from build123d import *

# Parameters (mm, degrees)
SKETCH2_R          = 6.57
CUT_EXTRUDE1_DEPTH = 10.189570175
SKETCH3_R          = 2.9
CUT_EXTRUDE2_DEPTH = 3.28
SKETCH4_R          = 0.9
CUT_EXTRUDE3_DEPTH = 11.034288305


with BuildPart() as part:
    # Sketch1 → Revolve1 (revolve)
    with BuildSketch(Plane.XY, mode=Mode.PRIVATE) as revolve1_sk:
        Polygon((0, 5.22), (0, 1), (2.72, 1), (2.72, 0.42), (4.45, 0.42), (4.45, 0), (6.07, 0), (6.07, 1.94), (2.4, 1.94), (2.4, 5.22), align=None)
    revolve(revolve1_sk.sketch.rotate(Axis((0, 5.22, 0), (0, -1, 0)), 180), axis=Axis((0, 5.22, 0), (0, -1, 0)))

    # Sketch2 → Cut-Extrude1 (cut, through all)
    with BuildSketch(Plane(origin=(0, 1.94, 0), x_dir=(1, 0, 0), z_dir=(0, 1, 0))):
        Circle(SKETCH2_R)
        Polygon((0, 6.07), (-0.459966954, 5.550975626), (-0.999089163, 5.987213112), (-1.367354163, 5.399559481), (-1.970925778, 5.741110657), (-2.237443515, 5.100857429), (-2.889000676, 5.33840567), (-3.046501241, 4.663017284), (-3.728271166, 4.790082892), (-3.772458354, 4.097982182), (-4.465844138, 4.11109914), (-4.395512637, 3.42116481), (-5.081600523, 3.31997532), (-4.898668794, 2.651026979), (-5.558744093, 2.438291228), (-5.268202036, 1.808576043), (-5.884259614, 1.490096907), (-5.49403246, 0.916791868), (-6.049267873, 0.501256627), (-5.57, 0), (-6.049267873, -0.501256627), (-5.49403246, -0.916791868), (-5.884259614, -1.490096907), (-5.268202036, -1.808576043), (-5.558744093, -2.438291228), (-4.898668794, -2.651026979), (-5.081600523, -3.31997532), (-4.395512637, -3.42116481), (-4.465844138, -4.11109914), (-3.772458354, -4.097982182), (-3.728271166, -4.790082892), (-3.046501241, -4.663017284), (-2.889000676, -5.33840567), (-2.237443515, -5.100857429), (-1.970925778, -5.741110657), (-1.367354163, -5.399559481), (-0.999089163, -5.987213112), (-0.459966954, -5.550975626), (0, -6.07), (0.459966954, -5.550975626), (0.999089163, -5.987213112), (1.367354163, -5.399559481), (1.970925778, -5.741110657), (2.237443515, -5.100857429), (2.889000676, -5.33840567), (3.046501241, -4.663017284), (3.728271166, -4.790082892), (3.772458354, -4.097982182), (4.465844138, -4.11109914), (4.395512637, -3.42116481), (5.081600523, -3.31997532), (4.898668794, -2.651026979), (5.558744093, -2.438291228), (5.268202036, -1.808576043), (5.884259614, -1.490096907), (5.49403246, -0.916791868), (6.049267873, -0.501256627), (5.57, 0), (6.049267873, 0.501256627), (5.49403246, 0.916791868), (5.884259614, 1.490096907), (5.268202036, 1.808576043), (5.558744093, 2.438291228), (4.898668794, 2.651026979), (5.081600523, 3.31997532), (4.395512637, 3.42116481), (4.465844138, 4.11109914), (3.772458354, 4.097982182), (3.728271166, 4.790082892), (3.046501241, 4.663017284), (2.889000676, 5.33840567), (2.237443515, 5.100857429), (1.970925778, 5.741110657), (1.367354163, 5.399559481), (0.999089163, 5.987213112), (0.459966954, 5.550975626), align=None, mode=Mode.SUBTRACT)
    extrude(amount=-CUT_EXTRUDE1_DEPTH, mode=Mode.SUBTRACT)

    # Sketch3 → Cut-Extrude2 (cut)
    with BuildSketch(Plane(origin=(0, 5.22, 0), x_dir=(1, 0, 0), z_dir=(0, 1, 0))):
        Circle(SKETCH3_R)
        Polygon((0, 2.4), (-0.463525492, 1.426584774), (-1.410684606, 1.941640786), (-1.213525492, 0.881677878), (-2.282535639, 0.741640786), (-1.5, 0), (-2.282535639, -0.741640786), (-1.213525492, -0.881677878), (-1.410684606, -1.941640786), (-0.463525492, -1.426584774), (0, -2.4), (0.463525492, -1.426584774), (1.410684606, -1.941640786), (1.213525492, -0.881677878), (2.282535639, -0.741640786), (1.5, 0), (2.282535639, 0.741640786), (1.213525492, 0.881677878), (1.410684606, 1.941640786), (0.463525492, 1.426584774), align=None, mode=Mode.SUBTRACT)
    extrude(amount=-CUT_EXTRUDE2_DEPTH, mode=Mode.SUBTRACT)

    # Sketch4 → Cut-Extrude3 (cut, through all)
    with BuildSketch(Plane(origin=(0, 5.22, 0), x_dir=(1, 0, 0), z_dir=(0, 1, 0))):
        with Locations(Location((0, 0, 0), (0, 0, 180))):
            Circle(SKETCH4_R)
    extrude(amount=-CUT_EXTRUDE3_DEPTH, mode=Mode.SUBTRACT)


solid = part.part
Design review of the part built by this model. Coordinates are the model's own, in mm. A direction names the side the tool comes from. Round coordinates to 2 decimals unless told otherwise and drop trailing zeros. Loops run counter-clockwise (first coordinate to the right, second up) from the corner with the lowest first, then second, coordinate; pieces in that order, holes last. Notation, with made-up numbers: (24, 74) - (41, 74) arc R25 ccw to (41, 92) - close; hole circle Ø11 at (-23, 75). An arc over 180 degrees is marked (long way). One line per item, written item: value. Start each with the question number.
1) Consider section D-D on x = 4.25. Give the boundary of the cut face in (y, z), then the cut area to 3 significant figures.
2) For faces 1 (the flat face through (0.93, 3.6, 1.68)), 2 (the flat face through (1.313, 3.603, 1.419)), 3 (the flat face through (0.235, 3.603, -1.906)), list the 3-axis set-ups (+Z, -Z, +X, -X, +Y, -Y) from which the entire face can be reached by the end or side of a thin tool; tool diameter is ignored.
3) To check wall thickness, follow L1, parallel to Y at x = -1.25, z = 1.25; L2, parallel to X at y = 1.05, z = 1; L3, parallel to Z at x = 4, y = 1.4. State the ranges of each line that lie inside material, in increasing order. Write a range as from..to.
4) Consider section A-A on y = 4.3. Give the boundary of the cut face in (x, z), then the cut area to 3 significant figures.
5) Consider section B-B on x = 0.75. Give the boundary of the cut face in (y, z), then the cut area to 3 significant figures.
6) Draft analysis for pull direction Z (two halves, no side actions). For faces 4 (the flat face through (-1, 5.22, -1)), 5 (the flat face through (0.23, 3.6, 1.92)), 6 (the flat face through (-0.23, 3.6, -1.92)), 7 (the flat face through (-1.31, 3.6, 1.4)), state which applies: +Z half, -Z half, draft (parallel to the pull), parting line (faces both ways), or undercut.
7) Insertion check: pin 1 Ø1.5 at (x, z) = (4, 3.5) entering from +Y; pin 2 Ø2 at (y, z) = (0.5, 0) entering from -X; pin 3 Ø1.5 at (x, z) = (3, -2) entering from -Y. Each pin has a flat end and moves straight along its axis. Give the tip position at first contact, or say it passes through.
8) Consider section C-C on x = -2.5. Give the boundary of the cut face in (y, z), then the cut area to 3 significant figures.
Reported:
1. outline: (0, -4.11) - (1.94, -4.11) - (1.94, 4.11) - (0, 4.11) - (0, 1.32) - (0.42, 1.32) - (0.42, -1.32) - (0, -1.32) - close
1. area: 14.8 mm^2
2. face 1: +Z, +Y
2. face 2: +X, +Y
2. face 3: -Z, +Y
3. L1: y = 1..5.22
3. L2: x = -5.55..5.55
3. L3: z = -4.1..4.1
4. outline: (-2.28, -0.74) - (-1.21, -0.88) - (-1.41, -1.94) - (-0.46, -1.43) - (0, -2.4) - (0.46, -1.43) - (1.41, -1.94) - (1.21, -0.88) - (2.28, -0.74) - (1.5, 0) - (2.28, 0.74) - (1.21, 0.88) - (1.41, 1.94) - (0.46, 1.43) - (0, 2.4) - (-0.46, 1.43) - (-1.41, 1.94) - (-1.21, 0.88) - (-2.28, 0.74) - (-1.5, 0) - close; hole circle Ø1.8 at (0, 0)
4. area: 8.58 mm^2
5. outline: (0, -5.79) - (1.94, -5.79) - (1.94, -1.58) - (5.22, -1.58) - (5.22, -0.5) - (1, -0.5) - (1, -2.61) - (0.42, -2.61) - (0.42, -4.39) - (0, -4.39) - close; (0, 4.39) - (0.42, 4.39) - (0.42, 2.61) - (1, 2.61) - (1, 0.5) - (5.22, 0.5) - (5.22, 1.58) - (1.94, 1.58) - (1.94, 5.79) - (0, 5.79) - close
5. area: 21.9 mm^2
6. face 4: draft
6. face 5: +Z half
6. face 6: -Z half
6. face 7: undercut
7. pin 1: stops at y = 1.94
7. pin 2: stops at x = -6.05
7. pin 3: stops at y = 0.42
8. outline: (0, -5.2) - (1.94, -5.2) - (1.94, 5.2) - (0, 5.2) - (0, 3.68) - (0.42, 3.68) - (0.42, 1.07) - (1, 1.07) - (1, -1.07) - (0.42, -1.07) - (0.42, -3.68) - (0, -3.68) - close
8. area: 15.8 mm^2
